```python
from build123d import *

# Parameters (mm, degrees)
SKETCH_1_W          = 60
SKETCH_1_H          = 108
EXTRUDE_1_DEPTH     = 1
SKETCH_2_R          = 1.6
CUT_EXTRUDE_1_DEPTH = 5
SKETCH_4_R          = 1.6
CUT_EXTRUDE_3_DEPTH = 5
FILLET_1_R          = 5
SKETCH_5_W          = 10
SKETCH_5_H          = 52
CUT_EXTRUDE_4_DEPTH = 62.781874365


with BuildPart() as part:
    # ｽｹｯﾁ1 → ﾎﾞｽ - 押し出し1 (new body)
    with BuildSketch(Plane.XY):
        Rectangle(SKETCH_1_W, SKETCH_1_H)
    extrude(amount=EXTRUDE_1_DEPTH)

    # ｽｹｯﾁ2 → ｶｯﾄ - 押し出し1 (cut)
    with BuildSketch(Plane.XY.offset(1)):
        with Locations((-3, 44)):
            Circle(SKETCH_2_R)
        with Locations((20, 44)):
            Circle(SKETCH_2_R)
        with Locations((-3, -14)):
            Circle(SKETCH_2_R)
        with Locations((20, -14)):
            Circle(SKETCH_2_R)
    extrude(amount=-CUT_EXTRUDE_1_DEPTH, mode=Mode.SUBTRACT)

    # ｽｹｯﾁ4 → ｶｯﾄ - 押し出し3 (cut)
    with BuildSketch(Plane.XY.offset(1)):
        with Locations((-25, 49)):
            Circle(SKETCH_4_R)
        with Locations((25, 49)):
            Circle(SKETCH_4_R)
        with Locations((-25, -49)):
            Circle(SKETCH_4_R)
        with Locations((25, -49)):
            Circle(SKETCH_4_R)
    extrude(amount=-CUT_EXTRUDE_3_DEPTH, mode=Mode.SUBTRACT)

    # ﾌｨﾚｯﾄ1
    fillet_1_edges = [part.edges().sort_by_distance(p)[0] for p in [
        (30, -54, 0.5),
        (-30, -54, 0.5),
        (-30, 54, 0.5),
        (30, 54, 0.5),
    ]]
    fillet(fillet_1_edges, radius=FILLET_1_R)

    # ｽｹｯﾁ5 → ｶｯﾄ - 押し出し4 (cut, through all)
    with BuildSketch(Plane(origin=(0, 0, 0), x_dir=(-1, 0, 0), z_dir=(0, 0, -1))):
        with Locations((-20, 15)):
            Rectangle(SKETCH_5_W, SKETCH_5_H)
    extrude(amount=-CUT_EXTRUDE_4_DEPTH, mode=Mode.SUBTRACT)


solid = part.part
```
The listing builds one solid part. Answer for the finished solid, in the listing's coordinates (mm). Give positions to 0.01 mm unless a question says otherwise; leave off trailing zeros. Order: outer loops, then holes, each group sorted by start corner. A loop starts at its lowest first (then second) coordinate and runs counter-clockwise, first axis right, second up. Notation, with made-up numbers: M -36,18 L 3,18 A29 cw 3,55 Z; hole C 44,72 d7. An arc over 180 degrees is marked long. Put each result on its own line as item: value. Start each with the question number.
Item 1: The part is cut by section B-B, the plane z = 0.4. State how many separate pieces and enclosed holes the cut face has, and give its area (3 significant figures).
Item 2: The part is cut by section D-D, the plane y = 44. Determine the outline of the cut face in (x, z).
Item 3: For a pull along Y with two mould halves and no side action, classify faces 1 (the face through (-26.18, 50.08, 0.51)), 2 (the face through (28.5, -52.57, 0.51)), 3 (the face through (-28.57, 52.5, 0.51)) as +Y half, -Y half, draft (parallel to the pull), parting line (faces both ways), or undercut.
Item 4: Find the intervals of material crossed by line 1 along Y through (x, z) = (20, 0.5); line 2 along Y through (x, z) = (-3, 0.4); line 3 along X through (y, z) = (-2.5, 0.1), in increasing order.
Item 5: The part is cut by section C-C, the plane y = -3. Determine the outline of the cut face in (x, z), and give its area (3 significant figures).
Item 6: A flat-ended cylindrical pin translates along its axis: P1, Ø3, axis at x = -25, y = -49, coming from the +Z side. Find the tip coordinate at first contact, or state that the pin passes through.
Item 7: The part is cut by section A-A, the plane x = 20. Determine the outline of the cut face in (y, z).
Answer key:
1. separate pieces: 1
1. enclosed holes: 9
1. area: 5,870 mm²
2. outline: M -30,0 L -4.6,0 L -4.6,1 L -30,1 Z; M -1.4,0 L 18.4,0 L 18.4,1 L -1.4,1 Z; M 21.6,0 L 30,0 L 30,1 L 21.6,1 Z
3. face 1: undercut
3. face 2: -Y half
3. face 3: +Y half
4. line 1: y = -54 to -15.6, -12.4 to -11, 41 to 42.4, 45.6 to 54
4. line 2: y = -54 to -15.6, -12.4 to 42.4, 45.6 to 54
4. line 3: x = -30 to 15, 25 to 30
5. outline: M -30,0 L 15,0 L 15,1 L -30,1 Z; M 25,0 L 30,0 L 30,1 L 25,1 Z
5. area: 50.0 mm²
6. P1: passes through
7. outline: M -54,0 L -15.6,0 L -15.6,1 L -54,1 Z; M -12.4,0 L -11,0 L -11,1 L -12.4,1 Z; M 41,0 L 42.4,0 L 42.4,1 L 41,1 Z; M 45.6,0 L 54,0 L 54,1 L 45.6,1 Z
